Can you work these out from the model? Positions are in its coordinate system, mm. Coordinates: 2 decimals unless noted, no trailing zeros. Order: outer loops, then holes, each group sorted by start corner. A loop starts at its lowest first (then second) coordinate and runs counter-clockwise, first axis right, second up. Notation, with made-up numbers: (-8.75, 23) - (12.25, 23) arc R16 ccw to (12.25, 31) - close; hole circle Ø10 at (-7.75, 6). An arc over 180 degrees is marked (long way). Use a Markdown table: item, result. Add a question column.
(1) I want a section at C-C (z = 1.6). State how many separate pieces and enclosed holes the cut face has, and give its area (3 significant figures).
(2) I want a section at A-A (y = 30). List the corners of the cut face in (x, z) for me.
(3) For pin 1 Ø8 at (x, y) = (112, 69.5) entering from -Z; pin 2 Ø2.5 at (x, y) = (129.54, 78.79) entering from -Z, each with a flat end and sliding along its axis, tell me the tip position at first contact or that it passes through.
(4) I want a section at B-B (x = 101.6). List the corners of the cut face in (y, z) for me.
(5) I want a section at D-D (x = 129.54). List the corners of the cut face in (y, z) for me.
(6) If I drill on L1, parallel to Y at x = 100.33, z = 3.8; L2, parallel to X at y = 87, z = 0.2; L3, parallel to X at y = 99, z = 4, over which ranges is the centre line in solid material (lowest first)? Write a range as [from, to].
```python
from build123d import *

# Parameters (mm, degrees)
SKETCH1_W           = 158.75
SKETCH1_H           = 114.3
SKETCH1_R           = 6.35
SKETCH1_R_2         = 1.5875
BOSS_EXTRUDE1_DEPTH = 4.7752
FILLET2_R           = 6.35
SKETCH2_R           = 6.35
CUT_EXTRUDE1_DEPTH  = 20.32


with BuildPart() as part:
    # Sketch1 → Boss-Extrude1 (new body)
    with BuildSketch(Plane.XY):
        with Locations((79.375, 57.15)):
            Rectangle(SKETCH1_W, SKETCH1_H)
        with Locations((101.6, 90.17)):
            Circle(SKETCH1_R, mode=Mode.SUBTRACT)
        with Locations((119.38, 79.233708435)):
            Circle(SKETCH1_R_2, mode=Mode.SUBTRACT)
        with Locations((129.54, 78.790113255)):
            Circle(SKETCH1_R_2, mode=Mode.SUBTRACT)
        with Locations((139.7, 78.346518075)):
            Circle(SKETCH1_R_2, mode=Mode.SUBTRACT)
        with BuildLine():
            ThreePointArc((122.551978104, 89.25521688), (122.492134184, 91.997824898), (122.074820056, 94.709158325))
            ThreePointArc((122.074820056, 94.709158325), (118.287884459, 97.121702373), (115.87534041, 93.334766776))
            ThreePointArc((115.87534041, 93.334766776), (116.166297851, 91.444385931), (116.208021896, 89.53219999))
            ThreePointArc((116.208021896, 89.53219999), (119.241508445, 86.221730332), (122.551978104, 89.25521688))
        make_face(mode=Mode.SUBTRACT)
        with BuildLine():
            ThreePointArc((142.871978104, 88.36802652), (142.754095346, 93.7705168), (141.932054608, 99.11140124))
            ThreePointArc((141.932054608, 99.11140124), (138.145119011, 101.523945288), (135.732574962, 97.737009691))
            ThreePointArc((135.732574962, 97.737009691), (136.428259013, 93.217077834), (136.528021896, 88.64500963))
            ThreePointArc((136.528021896, 88.64500963), (139.561508445, 85.334539972), (142.871978104, 88.36802652))
        make_face(mode=Mode.SUBTRACT)
        with BuildLine():
            ThreePointArc((132.711978104, 88.8116217), (132.623114765, 92.884170849), (132.003437332, 96.910279782))
            ThreePointArc((132.003437332, 96.910279782), (128.216501735, 99.322823831), (125.803957686, 95.535888234))
            ThreePointArc((125.803957686, 95.535888234), (126.297278432, 92.330731883), (126.368021896, 89.08860481))
            ThreePointArc((126.368021896, 89.08860481), (129.401508445, 85.778135152), (132.711978104, 88.8116217))
        make_face(mode=Mode.SUBTRACT)
    extrude(amount=BOSS_EXTRUDE1_DEPTH)

    # Fillet2
    fillet2_edges = [part.edges().sort_by_distance(p)[0] for p in [
        (0, 114.3, 2.3876),
        (158.75, 114.3, 2.3876),
        (158.75, 0, 2.3876),
        (0, 0, 2.3876),
    ]]
    fillet(fillet2_edges, radius=FILLET2_R)

    # Sketch2 → Cut-Extrude1 (cut)
    with BuildSketch(Plane.XY.offset(4.7752)):
        with Locations((100.33, 25.4)):
            Circle(SKETCH2_R)
    extrude(amount=-CUT_EXTRUDE1_DEPTH, mode=Mode.SUBTRACT)


solid = part.part
```
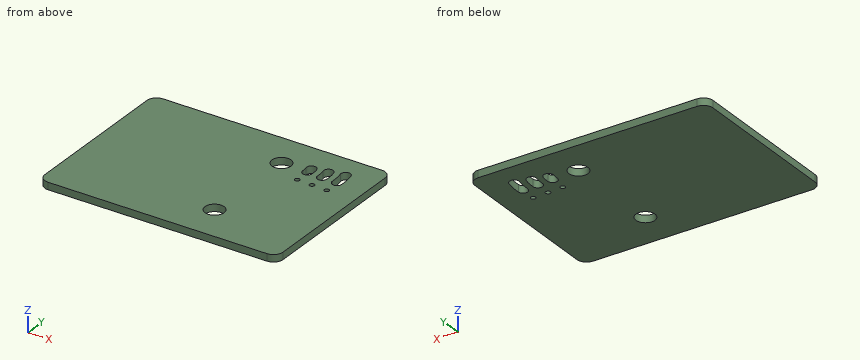
Answers follow:
| question | item | result |
|---|---|---|
| 1 | separate pieces | 1 |
| 1 | enclosed holes | 8 |
| 1 | area | 17,600 mm² |
| 2 | outline | (0, 0) - (95.95, 0) - (95.95, 4.78) - (0, 4.78) - close; (104.71, 0) - (158.75, 0) - (158.75, 4.78) - (104.71, 4.78) - close |
| 3 | pin 1 | stops at z = 0 |
| 3 | pin 2 | passes through |
| 4 | outline | (0, 0) - (19.18, 0) - (19.18, 4.78) - (0, 4.78) - close; (31.62, 0) - (83.82, 0) - (83.82, 4.78) - (31.62, 4.78) - close; (96.52, 0) - (114.3, 0) - (114.3, 4.78) - (96.52, 4.78) - close |
| 5 | outline | (0, 0) - (77.2, 0) - (77.2, 4.78) - (0, 4.78) - close; (80.38, 0) - (85.78, 0) - (85.78, 4.78) - (80.38, 4.78) - close; (99.33, 0) - (114.3, 0) - (114.3, 4.78) - (99.33, 4.78) - close |
| 6 | L1 | y = [0, 19.05], [31.75, 83.95], [96.39, 114.3] |
| 6 | L2 | x = [0, 96.1], [107.1, 117.29], [121.47, 127.03], [132.05, 136.91], [142.49, 158.75] |
| 6 | L3 | x = [0, 127.36], [130.44, 135.71], [141.96, 158.75] |
